```python
from build123d import *

# Parameters (mm, degrees)
F0_W        = 20
F0_H        = 14
F1_DEPTH    = 25
F3_D        = 5
F5_D        = 5
F6_T1_DEPTH = 44.999500005
F7_T1_DEPTH = 34.0317226184


# Not quite as in the source:
# - a fillet or chamfer that OpenCascade refuses, or shapes differently, is made with other operations: its cross-section is extruded or revolved along the edge and cut away or added


with BuildPart() as f1:
    # F0 (on Right) → F1 (new body, symmetric)
    with BuildSketch(Plane.YZ):
        Rectangle(F0_W, F0_H)
    extrude(amount=F1_DEPTH, both=True)

    # F3 (through all)
    with Locations(Plane.XZ.offset(10)):
        with Locations((4, 1), (20, 1)):
            Hole(F3_D / 2)

    # F5 (through all)
    with Locations(Plane.XY.offset(7)):
        with Locations((-16, 0), (14, 0)):
            Hole(F5_D / 2)

    # F6: fillet of radius 5 on 3 edges, made by hand

    # F6_s2 → F6_t1 (cut)
    with BuildSketch(Plane.XZ.offset(-22.4997500025)):
        with BuildLine():
            ThreePointArc((25.0001, 2.0001), (23.5356339059, 5.5356339059), (20.0001, 7.0001))
            Line((20.0001, 7.0001), (20.0001, 7.1001))
            ThreePointArc((20.0001, 7.1001), (22.50005, 7.1), (25, 7.1))
            Line((25, 7.1), (25.1, 7))
            ThreePointArc((25.1, 7), (25.1, 4.50005), (25.1001, 2.0001))
            Line((25.1001, 2.0001), (25.0001, 2.0001))
        make_face()
        with BuildLine():
            ThreePointArc((-20.0001, -7.0001), (-23.5356339059, -5.5356339059), (-25.0001, -2.0001))
            Line((-25.0001, -2.0001), (-25.1001, -2.0001))
            ThreePointArc((-25.1001, -2.0001), (-25.1, -4.50005), (-25.1, -7))
            Line((-25.1, -7), (-25, -7.1))
            ThreePointArc((-25, -7.1), (-22.50005, -7.1), (-20.0001, -7.1001))
            Line((-20.0001, -7.1001), (-20.0001, -7.0001))
        make_face()
        with BuildLine():
            ThreePointArc((20.0001, -7.0001), (23.5356339059, -5.5356339059), (25.0001, -2.0001))
            Line((25.0001, -2.0001), (25.1001, -2.0001))
            ThreePointArc((25.1001, -2.0001), (25.1, -4.50005), (25.1, -7))
            Line((25.1, -7), (25, -7.1))
            ThreePointArc((25, -7.1), (22.50005, -7.1), (20.0001, -7.1001))
            Line((20.0001, -7.1001), (20.0001, -7.0001))
        make_face()
    extrude(amount=F6_T1_DEPTH, mode=Mode.SUBTRACT)

    # F7: fillet of radius 5 on 1 edges, made by hand

    # F7_s2 → F7_t1 (cut)
    with BuildSketch(Plane.XY.offset(-14.5317226184)):
        with BuildLine():
            ThreePointArc((-20, -10), (-23.5355339059, -8.5355339059), (-25, -5))
            Line((-25, -5), (-25, -10))
            Line((-25, -10), (-20, -10))
        make_face()
    extrude(amount=F7_T1_DEPTH, mode=Mode.SUBTRACT)


solid = f1.part
```
Check sheet for the modelled part. Datum: model origin and axes. Units: mm. Give positions to 0.01 mm unless a question says otherwise; leave off trailing zeros. Write each loop counter-clockwise with the first axis right and the second up, starting at its lowest first coordinate (ties: lowest second). Pieces come first, ordered by that corner, then holes. Notation, with made-up numbers: (-33.75, 19) -> (7.25, 19) arc R11 ccw to (7.25, 34) -> close; hole circle Ø3 at (-27, -20.5). An arc over 180 degrees is marked (long way). Use CSV: the item, a comma, the result in double quotes. Start each with the question number.
Q1. Cross-section at C-C on z = 1. Enter the section's corners in (x, y).
Q2. Scan lines: line 1 along Y through (x, z) = (-16, 0); line 2 along Z through (x, y) = (4, 1.5); line 3 along Y through (x, z) = (-18, -1). Record each from-to range of solid material in increasing order.
Q3. Release check for a two-part mould opening along X. For faces 1 (the cylindrical face through (-13.5, 0.1, -0.1)), 2 (the cylindrical face through (24, 0, 5)), 3 (the flat face through (-25, 2, 3)), 4 (the cylindrical face through (1.615, 0.14, 1.751)) record: +X half, -X half, draft (parallel to the pull), parting line (faces both ways), or undercut.
Q4. Cross-section at A-A on y = -1.5. Enter the section's corners in (x, z).
Q5. Depth check by flat-ended pin: P1, Ø6.5, axis at x = 20, z = 1, coming from the -Y side. Enter the tip coordinate at first touch or a pass-through.
Q6. Cross-section at D-D on y = 4. Enter the section's corners in (x, z), and give its area (3 significant figures).
Q7. Cross-section at B-B on x = 18. Enter the section's corners in (y, z), and give its area (3 significant figures).
Working result:
1,outline,"(-25, -5) arc R5 ccw to (-20, -10) -> (1.5, -10) -> (1.5, 10) -> (-25, 10) -> close; (6.5, -10) -> (17.5, -10) -> (17.5, 10) -> (6.5, 10) -> close; (22.5, -10) -> (25, -10) -> (25, 10) -> (22.5, 10) -> close; hole circle Ø5 at (-16, 0); hole circle Ø5 at (14, 0)"
2,line 1,"y = -10 to -2.5, 2.5 to 10"
2,line 2,"z = -7 to -1.5, 3.5 to 7"
2,line 3,"y = -10 to -1.5, 1.5 to 10"
3,face 1,"undercut"
3,face 2,"+X half"
3,face 3,"-X half"
3,face 4,"undercut"
4,outline,"(-25, -2.03) arc R5 ccw to (-20.03, -7) -> (-18, -7) -> (-18, 7) -> (-25, 7) -> close; (-14, -7) -> (12, -7) -> (12, 7) -> (-14, 7) -> close; (16, -7) -> (20.03, -7) arc R5 ccw to (25, -2.03) -> (25, 2.03) arc R5 ccw to (20.03, 7) -> (16, 7) -> close; hole circle Ø5 at (4, 1); hole circle Ø5 at (20, 1)"
5,P1,"stops at y = -10"
6,outline,"(-25, -2.03) arc R5 ccw to (-20.03, -7) -> (20.03, -7) arc R5 ccw to (25, -2.03) -> (25, 2.03) arc R5 ccw to (20.03, 7) -> (-25, 7) -> close; hole circle Ø5 at (4, 1); hole circle Ø5 at (20, 1)"
6,area,"645 mm^2"
7,outline,"(-10, -7) -> (10, -7) -> (10, -0.5) -> (-10, -0.5) -> close; (-10, 2.5) -> (10, 2.5) -> (10, 7) -> (-10, 7) -> close"
7,area,"220 mm^2"
